Work out the finished part from the listing and answer in its coordinate system (mm). Face numbers are marked on the shaded views. A direction names the side the tool comes from. Coordinates: 2 decimals unless noted, no trailing zeros. Write each loop counter-clockwise with the first axis right and the second up, starting at its lowest first coordinate (ties: lowest second). Pieces come first, ordered by that corner, then holes. Notation, with made-up numbers: (41, -28.5) - (78, -28.5) arc R21 ccw to (78, -15.5) - close; hole circle Ø8 at (32, -19.5). An arc over 180 degrees is marked (long way). Answer as a JSON object with one key per item and string values. Group by question number.
from build123d import *

# Parameters (mm, degrees)
F1_DEPTH  = 25
F2_R      = 2
F3_R      = 2
F0_R      = 1.5
F4_DEPTH  = 2
F0_W      = 9.26834
F0_H      = 8.993458
F0_R_2    = 2.5
F5_DEPTH  = 19
F6_R      = 5
F0_R_3    = 1.6
F7_DEPTH  = 19
F8_DEPTH  = 10
F10_DEPTH = 25


with BuildPart() as f1:
    # F0 (on Top) → F1 (new body)
    with BuildSketch(Plane.XY):
        Polygon((-47.95, 31.5), (-47.95, 0), (-47.95, -31.5), (0, -31.5), (47.95, -31.5), (47.95, 0), (47.95, 31.5), (0, 31.5), align=None)
        Polygon((-46, -20.506542), (-46, 0), (-46, 20.506542), (-46, 29.5), (-36.73166, 29.5), (0, 29.5), (36.73166, 29.5), (46, 29.5), (46, 20.506542), (46, 0), (46, -20.506542), (46, -29.5), (36.73166, -29.5), (0, -29.5), (-36.73166, -29.5), (-46, -29.5), align=None, mode=Mode.SUBTRACT)
    extrude(amount=F1_DEPTH)

    # F2
    f2_edges = [f1.edges().sort_by_distance(p)[0] for p in [
        (-47.95, -31.5, 12.5),
    ]]
    fillet(f2_edges, radius=F2_R)

    # F3
    f3_edges = [f1.edges().sort_by_distance(p)[0] for p in [
        (47.95, -31.5, 12.5),
        (47.95, 31.5, 12.5),
        (-47.95, 31.5, 12.5),
    ]]
    fillet(f3_edges, radius=F3_R)

    # F0 (on Top) → F4 (join)
    with BuildSketch(Plane.XY):
        Polygon((-46, 20.506542), (-46, 0), (-46, -20.506542), (-36.73166, -20.506542), (-36.73166, -29.5), (0, -29.5), (36.73166, -29.5), (36.73166, -20.506542), (46, -20.506542), (46, 0), (46, 20.506542), (36.73166, 20.506542), (36.73166, 29.5), (0, 29.5), (-36.73166, 29.5), (-36.73166, 20.506542), align=None)
        with Locations((-26.690211, -17.429141)):
            Circle(F0_R, mode=Mode.SUBTRACT)
        with Locations((26.690211, -17.429141)):
            Circle(F0_R, mode=Mode.SUBTRACT)
        with Locations((-26.690211, 17.429141)):
            Circle(F0_R, mode=Mode.SUBTRACT)
        with Locations((26.690211, 17.429141)):
            Circle(F0_R, mode=Mode.SUBTRACT)
    extrude(amount=F4_DEPTH)

    # F0 (on Top) → F5 (join)
    with BuildSketch(Plane.XY):
        with Locations((-41.36583, 25.003271)):
            Rectangle(F0_W, F0_H)
        with Locations((-40.7, 24.7)):
            Circle(F0_R_2, mode=Mode.SUBTRACT)
        with Locations((41.36583, 25.003271)):
            Rectangle(F0_W, F0_H)
        with Locations((40.7, 24.7)):
            Circle(F0_R_2, mode=Mode.SUBTRACT)
        with Locations((41.36583, -25.003271)):
            Rectangle(F0_W, F0_H)
        with Locations((40.7, -24.7)):
            Circle(F0_R_2, mode=Mode.SUBTRACT)
        with Locations((-41.36583, -25.003271)):
            Rectangle(F0_W, F0_H)
        with Locations((-40.7, -24.7)):
            Circle(F0_R_2, mode=Mode.SUBTRACT)
    extrude(amount=F5_DEPTH)

    # F6
    f6_edges = [f1.edges().sort_by_distance(p)[0] for p in [
        (-36.73166, 20.506542, 10.5),
        (36.73166, 20.506542, 10.5),
        (36.73166, -20.506542, 10.5),
        (-36.73166, -20.506542, 10.5),
    ]]
    fillet(f6_edges, radius=F6_R)

    # F0 (on Top) → F7 (join)
    with BuildSketch(Plane.XY):
        with Locations((-40.7, 24.7)):
            Circle(F0_R_2)
        with Locations((-40.7, 24.7)):
            Circle(F0_R_3, mode=Mode.SUBTRACT)
        with Locations((40.7, 24.7)):
            Circle(F0_R_2)
        with Locations((40.7, 24.7)):
            Circle(F0_R_3, mode=Mode.SUBTRACT)
        with Locations((40.7, -24.7)):
            Circle(F0_R_2)
        with Locations((40.7, -24.7)):
            Circle(F0_R_3, mode=Mode.SUBTRACT)
        with Locations((-40.7, -24.7)):
            Circle(F0_R_2)
        with Locations((-40.7, -24.7)):
            Circle(F0_R_3, mode=Mode.SUBTRACT)
    extrude(amount=F7_DEPTH)

    # F0 (on Top) → F8 (cut)
    with BuildSketch(Plane.XY):
        with Locations((-40.7, 24.7)):
            Circle(F0_R_2)
        with Locations((-40.7, 24.7)):
            Circle(F0_R_3, mode=Mode.SUBTRACT)
        with Locations((-40.7, -24.7)):
            Circle(F0_R_2)
        with Locations((-40.7, -24.7)):
            Circle(F0_R_3, mode=Mode.SUBTRACT)
        with Locations((40.7, -24.7)):
            Circle(F0_R_2)
        with Locations((40.7, -24.7)):
            Circle(F0_R_3, mode=Mode.SUBTRACT)
        with Locations((40.7, 24.7)):
            Circle(F0_R_2)
        with Locations((40.7, 24.7)):
            Circle(F0_R_3, mode=Mode.SUBTRACT)
    extrude(amount=F8_DEPTH, mode=Mode.SUBTRACT)

    # F9 (on face) → F10 (cut)
    with BuildSketch(Plane.YZ.offset(47.95)):
        Polygon((-4, 4), (0, 4), (4, 4), (4, 7), (0, 7), (-4, 7), align=None)
    extrude(amount=-F10_DEPTH, mode=Mode.SUBTRACT)


solid = f1.part
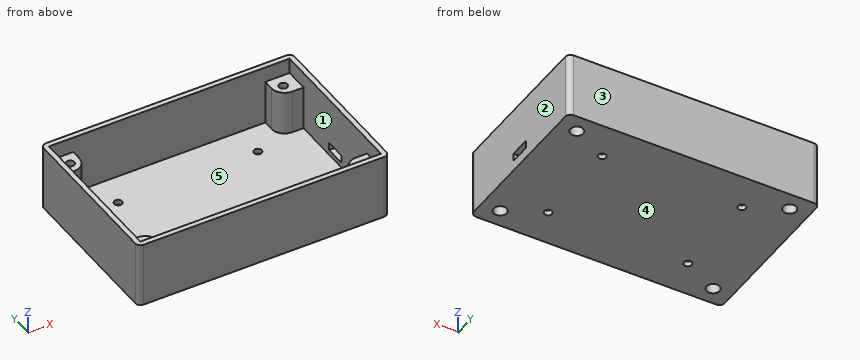
Q1. Consider L1, parallel to X at y = -14, z = 18.5; L2, parallel to Y at x = -17, z = 23.25; L3, parallel to Y at x = 40, z = 13.5. Determine where each line is inside the solid, lowest interval first. Write a range as from..to.
Q2. Section A-A on z = 21.25 is taken. Determine the outline of the cut face in (x, y).
Q3. For a pull along Y with two mould halves and no side action, classify the marked faces 1, 2 and 3 as +Y half, -Y half, draft (parallel to the pull), parting line (faces both ways), or undercut.
Q4. Section C-C on y = -8 is taken. Determine the outline of the cut face in (x, z), plus the area to 4 significant figures.
Q5. Section D-D on z = 5.75 is taken. Count the separate pieces of the cut face and the enclosed holes in it, plus the area to 3 significant figures.
Q6. Section B-B on x = -40.7 is taken. Determine the outline of the cut face in (y, z), plus the area to 3 significant figures.
Q7. A tool of negligible diameter and unlimited length cuts with its end or side. For the marked faces 4 and 5, from which of +Z, -Z, +X, -X, +Y, -Y can it reach the whole face along a straight path? Write none if from no direction.
Q8. Flat-ended cylindrical pins translate along their axes: pin 1 Ø4 at (x, y) = (19.5, 18.5) entering from +Z; pin 2 Ø1 at (x, z) = (47, 5.5) entering from +Y; pin 3 Ø3.5 at (x, y) = (-40.7, -24.7) entering from -Z; pin 4 Ø2.5 at (x, y) = (-40.7, 24.7) entering from +Z. Find the tip coordinate at first contact, or state that the pin passes through.
Numbers:
{
 "1": {"L1": "x = -47.95..-46, 46..47.95", "L2": "y = -31.5..-29.5, 29.5..31.5", "L3": "y = -31.5..-26.14, -23.26..-20.82, 20.82..23.26, 26.14..31.5"},
 "2": {"outline": "(-47.95, -29.5) arc R2 ccw to (-45.95, -31.5) - (45.95, -31.5) arc R2 ccw to (47.95, -29.5) - (47.95, 29.5) arc R2 ccw to (45.95, 31.5) - (-45.95, 31.5) arc R2 ccw to (-47.95, 29.5) - close; hole (-46, -29.5) - (46, -29.5) - (46, 29.5) - (-46, 29.5) - close"},
 "3": {"face 1": "undercut", "face 2": "draft", "face 3": "+Y half"},
 "4": {"outline": "(-47.95, 0) - (47.95, 0) - (47.95, 25) - (46, 25) - (46, 2) - (-46, 2) - (-46, 25) - (-47.95, 25) - close", "area": "281.5 mm²"},
 "5": {"separate pieces": "1", "enclosed holes": "4", "area": "828 mm²"},
 "6": {"outline": "(-31.5, 0) - (-27.2, 0) - (-27.2, 10) - (-26.3, 10) - (-26.3, 19) - (-29.5, 19) - (-29.5, 25) - (-31.5, 25) - close; (-23.1, 10) - (-22.2, 10) - (-22.2, 0) - (22.2, 0) - (22.2, 10) - (23.1, 10) - (23.1, 19) - (20.61, 19) - (20.61, 2) - (-20.61, 2) - (-20.61, 19) - (-23.1, 19) - close; (26.3, 10) - (27.2, 10) - (27.2, 0) - (31.5, 0) - (31.5, 25) - (29.5, 25) - (29.5, 19) - (26.3, 19) - close", "area": "363 mm²"},
 "7": {"face 4": "-Z, +X, -X, +Y, -Y", "face 5": "+Z"},
 "8": {"pin 1": "stops at z = 2", "pin 2": "stops at y = 31.42", "pin 3": "stops at z = 10", "pin 4": "passes through"}
}
